from build123d import *

# Parameters (mm, degrees)
SKETCH1_W           = 70
SKETCH1_H           = 20
BOSS_EXTRUDE1_DEPTH = 32
SKETCH3_R           = 1.2
CUT_EXTRUDE1_DEPTH  = 10
SKETCH3_3_R         = 0.6
CUT_EXTRUDE2_DEPTH  = 12
SKETCH3_4_R         = 0.6
CUT_EXTRUDE3_DEPTH  = 16
SKETCH3_5_R         = 0.6
CUT_EXTRUDE4_DEPTH  = 20
SKETCH3_6_R         = 0.6
CUT_EXTRUDE5_DEPTH  = 26
SKETCH4_R           = 2.5
SKETCH4_R_2         = 4
CUT_EXTRUDE6_DEPTH  = 15


with BuildPart() as part:
    # Sketch1 → Boss-Extrude1 (new body)
    with BuildSketch(Plane.XY):
        Rectangle(SKETCH1_W, SKETCH1_H)
    extrude(amount=BOSS_EXTRUDE1_DEPTH)

    # Sketch3 → Cut-Extrude1 (cut)
    with BuildSketch(Plane.XY.offset(32)):
        with Locations((28, 0)):
            Circle(SKETCH3_R)
    extrude(amount=-CUT_EXTRUDE1_DEPTH, mode=Mode.SUBTRACT)

    # Sketch3_3 → Cut-Extrude2 (cut)
    with BuildSketch(Plane.XY.offset(32)):
        with Locations((14, 0)):
            Circle(SKETCH3_3_R)
    extrude(amount=-CUT_EXTRUDE2_DEPTH, mode=Mode.SUBTRACT)

    # Sketch3_4 → Cut-Extrude3 (cut)
    with BuildSketch(Plane.XY.offset(32)):
        Circle(SKETCH3_4_R)
    extrude(amount=-CUT_EXTRUDE3_DEPTH, mode=Mode.SUBTRACT)

    # Sketch3_5 → Cut-Extrude4 (cut)
    with BuildSketch(Plane.XY.offset(32)):
        with Locations((-14, 0)):
            Circle(SKETCH3_5_R)
    extrude(amount=-CUT_EXTRUDE4_DEPTH, mode=Mode.SUBTRACT)

    # Sketch3_6 → Cut-Extrude5 (cut)
    with BuildSketch(Plane.XY.offset(32)):
        with Locations((-28, 0)):
            Circle(SKETCH3_6_R)
    extrude(amount=-CUT_EXTRUDE5_DEPTH, mode=Mode.SUBTRACT)

    # Sketch4 → Cut-Extrude6 (cut)
    with BuildSketch(Plane(origin=(0, 10, 0), x_dir=(1, 0, 0), z_dir=(0, 1, 0))):
        with Locations((28, -24.5)):
            Circle(SKETCH4_R)
        with Locations((14, -24)):
            Circle(SKETCH4_R_2)
        with Locations((0, -20)):
            Circle(SKETCH4_R_2)
        with Locations((-14, -16)):
            Circle(SKETCH4_R_2)
        with Locations((-28, -10)):
            Circle(SKETCH4_R_2)
    extrude(amount=-CUT_EXTRUDE6_DEPTH, mode=Mode.SUBTRACT)


solid = part.part
Verification items for the finished model (mm, model axes). A direction names the side the tool comes from. Give positions to 0.01 mm unless a question says otherwise; leave off trailing zeros. Write each loop counter-clockwise with the first axis right and the second up, starting at its lowest first coordinate (ties: lowest second). Pieces come first, ordered by that corner, then holes. Notation, with made-up numbers: (-26.75, 21.25) -> (-18.75, 21.25) arc R23 cw to (-18.75, 48.25) -> close; hole circle Ø1 at (53.5, 18.25). An arc over 180 degrees is marked (long way). Use CSV: the item, a comma, the result in double quotes.
(1) Go/stop test with flat-tipped pins: pin 1 (4 mm diameter, centred on x = 14.5, z = 22.5, fed in from +Y); pin 2 (1.1 mm diameter, centred on x = 0, y = 0, fed in from +Z). Record where each tip stops, or that it passes through.
Derived:
pin 1,"stops at y = -5"
pin 2,"stops at z = 16"
(2) Material ranges on L1, parallel to X at y = 0, z = 29.5; L2, parallel to Y at x = -28, z = 16; L3, parallel to Z at x = 14, y = 3, recorded low to high.
Derived:
L1,"x = -35 to -28.6, -27.4 to -14.6, -13.4 to -0.6, 0.6 to 13.4, 14.6 to 26.8, 29.2 to 35"
L2,"y = -10 to -0.6, 0.6 to 10"
L3,"z = 0 to 20, 28 to 32"
(3) Sectioned sample at C-C (z = 21). Record the cut outline in (x, y), plus the area to 3 significant figures.
Derived:
outline,"(-35, -10) -> (35, -10) -> (35, 10) -> (16.65, 10) -> (16.65, -5) -> (11.35, -5) -> (11.35, 10) -> (3.87, 10) -> (3.87, -5) -> (-3.87, -5) -> (-3.87, 10) -> (-35, 10) -> close; hole circle Ø1.2 at (-28, 0); hole circle Ø1.2 at (-14, 0)"
area,"1,200 mm^2"
(4) Sectioned sample at D-D (x = -16). Record the cut outline in (y, z), plus the area to 3 significant figures.
Derived:
outline,"(-10, 0) -> (10, 0) -> (10, 12.54) -> (-5, 12.54) -> (-5, 19.46) -> (10, 19.46) -> (10, 32) -> (-10, 32) -> close"
area,"536 mm^2"
(5) Sectioned sample at B-B (z = 10). Record the cut outline in (x, y), plus the area to 3 significant figures.
Derived:
outline,"(-35, -10) -> (35, -10) -> (35, 10) -> (-24, 10) -> (-24, -5) -> (-32, -5) -> (-32, 10) -> (-35, 10) -> close"
area,"1,280 mm^2"
(6) Set-up check for faces 4 (the cylindrical face through (-31.2, 2.6, 12.4)), 5 (the flat face through (28, 0, 22)), 6 (the flat face through (-0.5, 10, 15.8)), 7 (the flat face through (35, 0, 16)): record each of +Z, -Z, +X, -X, +Y, -Y from which the full face is reachable in a straight line by a thin tool's end or side.
Derived:
face 4,"+Y"
face 5,"+Z"
face 6,"+Z, -Z, +X, -X, +Y"
face 7,"+Z, -Z, +X, +Y, -Y"
(7) Release check for a two-part mould opening along Z. For faces 1 (the flat face through (14, 0, 20)), 2 (the flat face through (-28, -5, 10)), 3 (the cylindrical face through (-13.446, -0.23, 26.062)) record: +Z half, -Z half, draft (parallel to the pull), parting line (faces both ways), or undercut.
Derived:
face 1,"+Z half"
face 2,"undercut"
face 3,"draft"
(8) Sectioned sample at A-A (y = 8). Record the cut outline in (x, z).
Derived:
outline,"(-35, 0) -> (35, 0) -> (35, 32) -> (-35, 32) -> close; hole circle Ø8 at (-28, 10); hole circle Ø8 at (-14, 16); hole circle Ø8 at (0, 20); hole circle Ø8 at (14, 24); hole circle Ø5 at (28, 24.5)"
